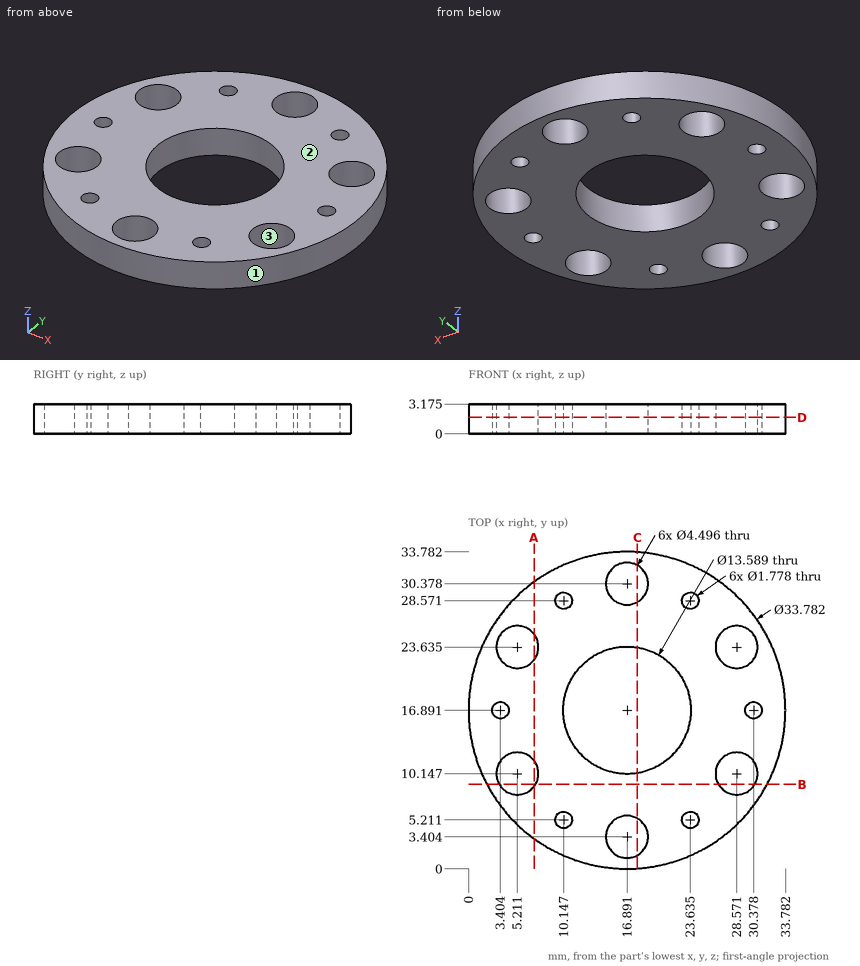
Geometry: see drawing. Coordinates: mm, zero at the bounding-box minimum. Coordinates: 2 decimals unless noted, no trailing zeros. Order: outer loops, then holes, each group sorted by start corner. A loop starts at its lowest first (then second) coordinate and runs counter-clockwise, first axis right, second up. Notation, with made-up numbers: M 6,-26 L 31,-26 A32 ccw 31,6 Z; hole C 82,1 d7. An arc over 180 degrees is marked long. Write each question's results on one line, items separated by ' | '. Start each with the question number.
1) Line query: line 1 (Y direction, x = 17, z = 1.6) (1 decimal); line 2 (X direction, y = 4.5, z = 1.35) (1 decimal); line 3 (X direction, y = 17, z = 1.5) (1 decimal). Output: solid intervals per line, ascending. Write a range as from..to.
2) Contact query for flat-ended pins moving along their axis: pin 1 Ø12 at (x, y) = (11, 8) entering from -Z; pin 2 Ø1 at (x, z) = (14, 2.5) entering from -Y. Output: stop coordinate, or through.
3) Section query B-B (y = 9). Return the cut outline in (x, z) (1 decimal).
4) Section query A-A (x = 7). Return the cut outline in (y, z) (1 decimal).
5) Section query C-C (x = 18). Return the cut outline in (y, z) (1 decimal).
6) Draft query along Y for the marked faces 1, 2 and 3. Return one class per face: released by +Y, released by -Y, zero draft, split by the parting line, or undercut.
7) Section query D-D (z = 1.75). Give the number of separate pieces and of enclosed holes in the cut face, plus the area to 3 significant figures.
Answers:
1) line 1: y = 0..1.2, 5.6..10.1, 23.7..28.1, 32.6..33.8 | line 2: x = 5.4..9.6, 10.7..14.9, 18.9..23.1, 24.2..28.4 | line 3: x = 0..2.5, 4.3..10.1, 23.7..29.5, 31.3..33.8
2) pin 1: stops at z = 0 | pin 2: stops at y = 0.17
3) outline: M 2,0 L 3.3,0 L 3.3,3.2 L 2,3.2 Z; M 7.1,0 L 26.6,0 L 26.6,3.2 L 7.1,3.2 Z; M 30.5,0 L 31.8,0 L 31.8,3.2 L 30.5,3.2 Z
4) outline: M 3.2,0 L 8.8,0 L 8.8,3.2 L 3.2,3.2 Z; M 11.5,0 L 22.3,0 L 22.3,3.2 L 11.5,3.2 Z; M 25,0 L 30.6,0 L 30.6,3.2 L 25,3.2 Z
5) outline: M 0,0 L 1.4,0 L 1.4,3.2 L 0,3.2 Z; M 5.4,0 L 10.2,0 L 10.2,3.2 L 5.4,3.2 Z; M 23.6,0 L 28.4,0 L 28.4,3.2 L 23.6,3.2 Z; M 32.3,0 L 33.7,0 L 33.7,3.2 L 32.3,3.2 Z
6) face 1: split by the parting line | face 2: zero draft | face 3: undercut
7) separate pieces: 1 | enclosed holes: 13 | area: 641 mm^2
